Could you check a few things on this drawing? It's one solid part, dimensions in mm from its lowest x, y, z. A direction names the side the tool comes from. Give positions to 0.01 mm unless a question says otherwise; leave off trailing zeros. Write each loop counter-clockwise with the first axis right and the second up, starting at its lowest first coordinate (ties: lowest second). Pieces come first, ordered by that corner, then holes. Notation, with made-up numbers: (52, -15.75) -> (65, -15.75) arc R11 ccw to (65, 0.25) -> close; hole circle Ø11 at (84.5, 59.25). An arc over 180 degrees is marked (long way). Use CSV: the item, a comma, the result in double quotes. Start each with the question number.
(1) Which directions (+Z, -Z, +X, -X, +Y, -Y) give clear straight access to the entire face, cutting with the end or side of a thin tool? Please do the marked faces 1 and 2.
(2) Suppose I cut it at B-B on z = 0.4. List the corners of the cut face in (x, y) for me, plus the area to 3 significant figures.
(3) I need wall thicknesses on L1, parallel to X at y = 3.05, z = 3.95; L2, parallel to Y at x = 6.5, z = 3.7. Which ranges of each line are inside material? Lowest first, please. Write a range as [from, to].
(4) Suppose I cut it at A-A on y = 2.1. List the corners of the cut face in (x, z) for me.
(5) For pin 1 Ø0.8 at (x, z) = (34, 2.5) entering from +Y, with a flat end and sliding along its axis, tell me the tip position at first contact or that it passes through.
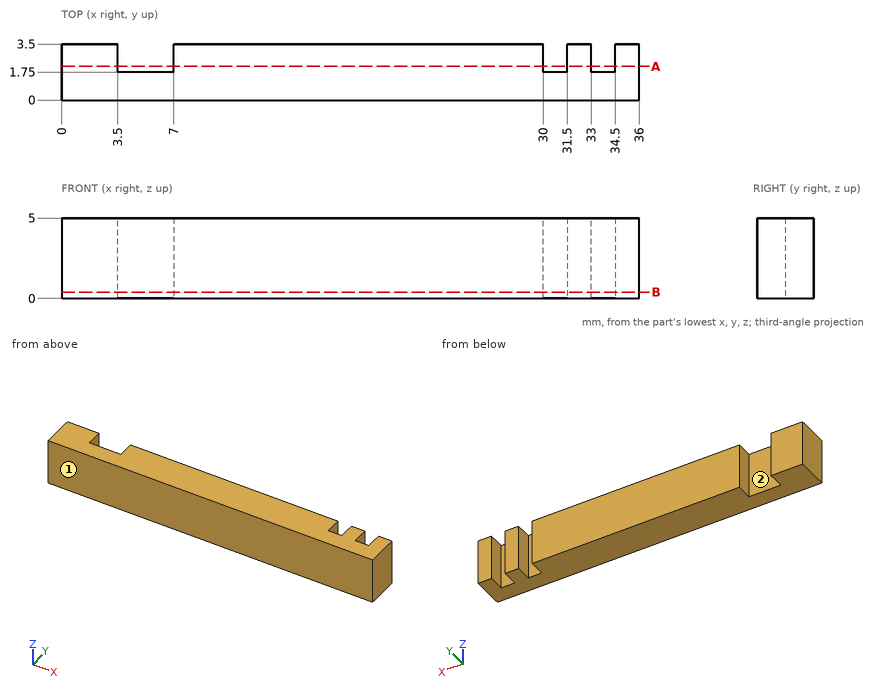
Geometry says:
1,face 1,"+Z, -Z, +X, -X, -Y"
1,face 2,"+Z, -Z, +Y"
2,outline,"(0, 0) -> (36, 0) -> (36, 3.5) -> (34.5, 3.5) -> (34.5, 1.75) -> (33, 1.75) -> (33, 3.5) -> (31.5, 3.5) -> (31.5, 1.75) -> (30, 1.75) -> (30, 3.5) -> (7, 3.5) -> (7, 1.75) -> (3.5, 1.75) -> (3.5, 3.5) -> (0, 3.5) -> close"
2,area,"115 mm²"
3,L1,"[0, 3.5], [7, 30], [31.5, 33], [34.5, 36]"
3,L2,"[0, 1.75]"
4,outline,"(0, 0) -> (3.5, 0) -> (3.5, 5) -> (0, 5) -> close; (7, 0) -> (30, 0) -> (30, 5) -> (7, 5) -> close; (31.5, 0) -> (33, 0) -> (33, 5) -> (31.5, 5) -> close; (34.5, 0) -> (36, 0) -> (36, 5) -> (34.5, 5) -> close"
5,pin 1,"y = 1.75"
